Could you check a few things on this model? Use its own coordinates, in mm. A direction names the side the tool comes from. Give positions to 0.01 mm unless a question says otherwise; leave off trailing zeros. Loops run counter-clockwise (first coordinate to the right, second up) from the corner with the lowest first, then second, coordinate; pieces in that order, holes last. Notation, with made-up numbers: M -12.5,-12 L -4.5,-12 A37 cw -4.5,24 Z; hole C -23,-0.5 d2. An arc over 180 degrees is marked long. Use a Markdown table: item, result. Add a question column.
1) Suppose I cut it at D-D on z = 30.25. List the corners of the cut face in (x, y) for me (3 decimals).
2) Suppose I cut it at C-C on y = -9. List the corners of the cut face in (x, z) for me, and give its area (3 significant figures).
3) If I drill on line 1 along Y through (x, z) = (-24.75, 9.5) (3 decimals); line 2 along Y through (x, z) = (24.75, 13) (3 decimals); line 3 along Z through (x, y) = (30, 1), over which ranges is the centre line in solid material (lowest first)? Write a range as [from, to].
4) We'd pull the mould along Y, two halves only. Please class faces 1 (the flat face through (-30.75, 0, 10)), 2 (the cylindrical face through (26.567, -4.428, 10.481)), 3 (the flat face through (-1, -13.425, 10)): +Y half, -Y half, draft (parallel to the pull), parting line (faces both ways), or undercut.
5) Will these pins go through, and if not, where does the flat tip stop? pin 1 Ø3 at (y, z) = (8, 9.5) entering from +X; pin 2 Ø10 at (x, y) = (65, 1) entering from -Z; pin 3 Ø8 at (y, z) = (-9, 9.5) entering from +X.
6) Suppose I cut it at B-B on y = 5. Count the separate pieces of the cut face and the enclosed holes in it, and give its area (3 significant figures).
7) Which directions (+Z, -Z, +X, -X, +Y, -Y) give clear straight access to the entire face, cutting with the end or side of a thin tool? Please do faces 4 (the flat face through (44, -7.075, 22)), 5 (the cylindrical face through (66.31, 5.26, 29.57)), 6 (the flat face through (20.5, 0, 10)).
```python
from build123d import *

# Parameters (mm, degrees)
BOSS_EXTRUDE1_DEPTH      = 15.1765
SKETCH3_W                = 41
SKETCH3_H                = 20.5
CUT_EXTRUDE1_DEPTH       = 27.178
SKETCH4_R                = 1.905
CUT_EXTRUDE2_DEPTH       = 12.7
SKETCH5_W                = 6.35
SKETCH5_H                = 9.525
CUT_EXTRUDE3_DEPTH       = 10.25
BOSS_EXTRUDE2_DEPTH      = 17.526
BOSS_EXTRUDE2_DEPTH_BACK = 1.5875
SKETCH7_W                = 38.1
SKETCH7_H                = 14.15
SKETCH7_R                = 1.016
FILLET3_R                = 15.875
FILLET4_R                = 6.35
CUT_EXTRUDE4_DEPTH       = 79.37799596
SKETCH11_W               = 161.059050972
SKETCH11_H               = 91.650514338
CUT_EXTRUDE5_DEPTH       = 20.828


with BuildPart() as part:
    # Sketch2 → Boss-Extrude1 (new, symmetric)
    with BuildSketch(Plane.XY):
        with BuildLine():
            Line((23.765883374, 13.425), (-24.4, 13.425))
            ThreePointArc((-24.4, 13.425), (-28.890128061, 11.565128061), (-30.75, 7.075))
            Line((-30.75, 7.075), (-30.75, -7.075))
            ThreePointArc((-30.75, -7.075), (-28.890128061, -11.565128061), (-24.4, -13.425))
            Line((-24.4, -13.425), (23.765883374, -13.425))
            ThreePointArc((23.765883374, -13.425), (28.256011435, -11.565128061), (30.115883374, -7.075))
            Line((30.115883374, -7.075), (30.115883374, 7.075))
            ThreePointArc((30.115883374, 7.075), (28.256011435, 11.565128061), (23.765883374, 13.425))
        make_face()
    extrude(amount=BOSS_EXTRUDE1_DEPTH, both=True)

    # Sketch3 → Cut-Extrude1 (cut)
    with BuildSketch(Plane.XY.offset(15.1765)):
        Rectangle(SKETCH3_W, SKETCH3_H)
    extrude(amount=-CUT_EXTRUDE1_DEPTH, mode=Mode.SUBTRACT)

    # Sketch4 → Cut-Extrude2 (cut)
    with BuildSketch(Plane.XY.offset(15.1765)):
        with Locations((-24.75, 5)):
            Circle(SKETCH4_R)
        with Locations((-24.75, -5)):
            Circle(SKETCH4_R)
        with Locations((24.75, -5)):
            Circle(SKETCH4_R)
        with Locations((24.75, 5)):
            Circle(SKETCH4_R)
    extrude(amount=-CUT_EXTRUDE2_DEPTH, mode=Mode.SUBTRACT)

    # Sketch5 → Cut-Extrude3 (cut)
    with BuildSketch(Plane.ZY.offset(30.75)):
        with Locations((-7.1755, 0)):
            Rectangle(SKETCH5_W, SKETCH5_H)
    extrude(amount=-CUT_EXTRUDE3_DEPTH, mode=Mode.SUBTRACT)


with BuildPart() as body_2:
    # Sketch7 → Boss-Extrude2 (new, two sides: drawn at the far end of the back side and taken through both)
    with BuildSketch(Plane.XY.offset(15.1765).offset(-BOSS_EXTRUDE2_DEPTH_BACK)):
        with Locations((49.165883374, 0)):
            Rectangle(SKETCH7_W, SKETCH7_H)
        with Locations((65.040883374, 0)):
            Circle(SKETCH7_R, mode=Mode.SUBTRACT)
        with Locations((58.690883374, 0)):
            Circle(SKETCH7_R, mode=Mode.SUBTRACT)
    extrude(amount=BOSS_EXTRUDE2_DEPTH + BOSS_EXTRUDE2_DEPTH_BACK)

    # Combine1: union part
    add(part.part)

    # Fillet3
    # the kernel refuses this fillet: 15.875 mm, written as the material it adds along each edge
    with BuildSketch(Plane(origin=(30.115883374, -7.075, 13.589), x_dir=(1, 0, 0), z_dir=(0, 1, 0))) as fillet3_piece_1:
        with BuildLine():
            CenterArc((FILLET3_R, FILLET3_R), FILLET3_R, 180, 90)
            Line((0, FILLET3_R), (0, 0))
            Line((0, 0), (FILLET3_R, 0))
        make_face()
    extrude(amount=14.15)

    # Fillet4
    fillet4_edges = [body_2.edges().sort_by_distance(p)[0] for p in [
        (68.215883374, -7.075, 23.14575),
        (68.215883374, 7.075, 23.14575),
    ]]
    fillet(fillet4_edges, radius=FILLET4_R)

    # Sketch9 → Cut-Extrude4 (cut, through all)
    with BuildSketch(Plane(origin=(0, 7.075, 0), x_dir=(1, 0, 0), z_dir=(0, 1, 0))):
        with BuildLine():
            Line((54.264591911, -32.7025), (24.88975776, -36.85029523))
            Line((24.88975776, -36.85029523), (30.115883374, -15.1765))
            ThreePointArc((30.115883374, -15.1765), (33.845663864, -16.387313537), (36.153060508, -19.558))
            ThreePointArc((36.153060508, -19.558), (43.075250443, -29.070059389), (54.264591911, -32.7025))
        make_face()
        with BuildLine():
            Line((59.502916407, -4.726647085), (70.262240595, -12.045992063))
            Line((70.262240595, -12.045992063), (68.215883374, -26.3525))
            Line((68.215883374, -26.3525), (55.515883374, -26.3525))
            ThreePointArc((55.515883374, -26.3525), (48.256026462, -24.072887594), (43.6024152, -18.052417734))
            ThreePointArc((43.6024152, -18.052417734), (41.400812879, -14.268836115), (38.045363181, -11.457519704))
            Line((38.045363181, -11.457519704), (42.798116213, -7.288485815))
            Line((42.798116213, -7.288485815), (59.502916407, -4.726647085))
        make_face()
    extrude(amount=-CUT_EXTRUDE4_DEPTH, mode=Mode.SUBTRACT)

    # Sketch11 → Cut-Extrude5 (cut)
    with BuildSketch(Plane(origin=(0, 0, -15.1765), x_dir=(-1, 0, 0), z_dir=(0, 0, -1))):
        Rectangle(SKETCH11_W, SKETCH11_H)
    extrude(amount=-CUT_EXTRUDE5_DEPTH, mode=Mode.SUBTRACT)


solid = body_2.part
```
Answer block:
| question | item | result |
|---|---|---|
| 1 | outline | M 44.914,-7.075 L 61.866,-7.075 A6.35 ccw 68.216,-0.725 L 68.216,0.725 A6.35 ccw 61.866,7.075 L 44.914,7.075 Z; hole C 58.691,0 d2.032; hole C 65.041,0 d2.032 |
| 2 | outline | M -30.45,5.65 L -20.5,5.65 L -20.5,15.18 L -30.45,15.18 Z; M 20.5,5.65 L 29.82,5.65 L 29.82,15.18 L 20.5,15.18 Z |
| 2 | area | 184 mm^2 |
| 3 | line 1 | y = [-13.415, -6.905], [-3.095, 3.095], [6.905, 13.415] |
| 3 | line 2 | y = [-13.348, -6.905], [-3.095, 3.095], [6.905, 13.348] |
| 3 | line 3 | z = [5.65, 15.18] |
| 4 | face 1 | draft |
| 4 | face 2 | undercut |
| 4 | face 3 | -Y half |
| 5 | pin 1 | stops at x = 36.83 |
| 5 | pin 2 | stops at z = 26.35 |
| 5 | pin 3 | stops at x = 40.18 |
| 6 | separate pieces | 4 |
| 6 | enclosed holes | 0 |
| 6 | area | 426 mm^2 |
| 7 | face 4 | +Z, -Z, +X, -Y |
| 7 | face 5 | +Z, -Z, +X, +Y |
| 7 | face 6 | +Z, -Z |
